Geometry: final body of the model. Coordinates: model frame, mm. Face numbers are marked on the shaded views. A direction names the side the tool comes from. Give positions to 0.01 mm unless a question says otherwise; leave off trailing zeros. Loops run counter-clockwise (first coordinate to the right, second up) from the corner with the lowest first, then second, coordinate; pieces in that order, holes last.
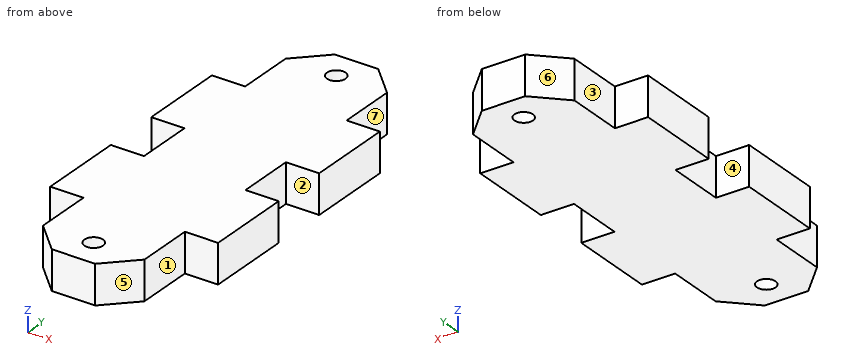
Autodesk Inventor part; units mm, degrees
ref_plane "YZ Plane" through (0, 0, 0) normal (1, 0, 0) x (0, 1, 0)
ref_plane "XZ Plane" through (0, 0, 0) normal (0, 1, 0) x (-1, 0, 0)
ref_plane "XY Plane" through (0, 0, 0) normal (0, 0, 1) x (1, 0, 0)
sketch "Sketch1" plane through (0, 0, 0) normal (0, 0, 1) x (1, 0, 0)
  line L0 (0, 0) -> (17.5, 0)
  line L1 (17.5, 0) -> (17.5, 70)
  line L2 (17.5, 70) -> (0, 70)
  line L3 (0, 70) -> (0, 0)
  line L4 (0, 55) -> (-5.731, 55)
  line L5 (-5.731, 55) -> (-5.731, 40)
  line L6 (-5.731, 40) -> (0, 40)
  line L7 (0, 40) -> (0, 55)
  line L8 (0, 30) -> (-5.731, 30)
  line L9 (-5.731, 30) -> (-5.731, 15)
  line L10 (-5.731, 15) -> (0, 15)
  line L11 (0, 15) -> (0, 30)
  circle A0 centre (8.75, 65) radius 1.6
  circle A1 centre (8.75, 5) radius 1.6
  line L12 (17.5, 55) -> (23.231, 55)
  line L13 (23.231, 55) -> (23.231, 40)
  line L14 (23.231, 40) -> (17.5, 40)
  line L15 (17.5, 40) -> (17.5, 55)
  line L16 (17.5, 30) -> (23.231, 30)
  line L17 (23.231, 30) -> (23.231, 15)
  line L18 (23.231, 15) -> (17.5, 15)
  line L19 (17.5, 15) -> (17.5, 30)
  point P0 (8.75, 70)
  dimension "d0" = 17.5
  dimension "d1" = 70
  dimension "d2" = 15
  dimension "d3" = 5.731
  dimension "d4" = 10
  dimension "d5" = 15
  dimension "d6" = 15
  dimension "d7" = 3.2
  dimension "d8" = 5
  dimension "d9" = 5
extrude "Extrusion1" add sketch "Sketch1" along normal blind 6.731
chamfer "Chamfer1" distance 5 angle 45 4 edges at (0, 70, 3.3655) (17.5, 70, 3.3655) (0, 0, 3.3655) (17.5, 0, 3.3655)
equation "\"d5\" = d6"
equation "\"d9\" = d8"
equation "\"d10\" = THICKB"
equation "\"THICKA\" = 3.175"
equation "\"THICKB\" = 6.731"
equation "\"THICKC\" = 12.7"
equation "\"MAGDIA\" = 9.5"
equation "\"BALLDIA\" = 12"
properties part number "Air2D_Bottom"
Item 1: Section query C-C on y = 11.5. Return loops of the section in (x, z), plus the area to 3 significant figures.
Values follow:
outline: (0, 0) - (17.5, 0) - (17.5, 6.73) - (0, 6.73) - close
area: 118 mm2
Item 2: Set-up query: the marked faces 1, 2 and 3. Return all of +Z, -Z, +X, -X, +Y, -Y with unobstructed straight access to the full face (end or side cutting, diameter ignored); none if empty.
Values follow:
face 1: +Z, -Z, +X, -Y
face 2: +Z, -Z, +X
face 3: +Z, -Z, -X, +Y
Item 3: Section query A-A on x = 8.75. Return loops of the section in (y, z), plus the area to 3 significant figures.
Values follow:
outline: (0, 0) - (3.4, 0) - (3.4, 6.73) - (0, 6.73) - close; (6.6, 0) - (63.4, 0) - (63.4, 6.73) - (6.6, 6.73) - close; (66.6, 0) - (70, 0) - (70, 6.73) - (66.6, 6.73) - close
area: 428 mm2
Item 4: Section query D-D on x = 15. Return loops of the section in (y, z), plus the area to 3 significant figures.
Values follow:
outline: (2.5, 0) - (67.5, 0) - (67.5, 6.73) - (2.5, 6.73) - close
area: 438 mm2
Item 5: Draft query along Y for the marked faces 4, 5, 6 and 7. Return one class per face: +Y half, -Y half, draft (parallel to the pull), parting line (faces both ways), or undercut.
Values follow:
face 4: undercut
face 5: -Y half
face 6: +Y half
face 7: draft
Item 6: Ray query, probe 1 along Y at (x, z) = (8.75, 1.75); probe 2 along X at (y, z) = (65, 3); probe 3 along Y at (x, z) = (-1.75, 4). Return the intervals inside material, ascending.
Values follow:
probe 1: y = 0 to 3.4, 6.6 to 63.4, 66.6 to 70
probe 2: x = 0 to 7.15, 10.35 to 17.5
probe 3: y = 15 to 30, 40 to 55
Item 7: Section query B-B on z = 3.5. Return loops of the section in (x, y), plus the area to 3 significant figures.
Values follow:
outline: (-5.73, 15) - (0, 15) - (0, 5) - (5, 0) - (12.5, 0) - (17.5, 5) - (17.5, 15) - (23.23, 15) - (23.23, 30) - (17.5, 30) - (17.5, 40) - (23.23, 40) - (23.23, 55) - (17.5, 55) - (17.5, 65) - (12.5, 70) - (5, 70) - (0, 65) - (0, 55) - (-5.73, 55) - (-5.73, 40) - (0, 40) - (0, 30) - (-5.73, 30) - close; hole circle Ø3.2 at (8.75, 5); hole circle Ø3.2 at (8.75, 65)
area: 1,500 mm2
Item 8: Pin query (flat end, axial travel): pin 1 (1.7 mm diameter, centred on x = -2, z = 4.5, fed in from -Y); pin 2 (1.7 mm diameter, centred on x = -1.5, z = 4, fed in from +Y); pin 3 (2 mm diameter, centred on y = 33.5, z = 4.5, fed in from -X); pin 4 (2.5 mm diameter, centred on x = 8.75, y = 5, fed in from -Z). Return the tip coordinate at first contact, or that it passes through.
Values follow:
pin 1: stops at y = 15
pin 2: stops at y = 55
pin 3: stops at x = 0
pin 4: passes through
